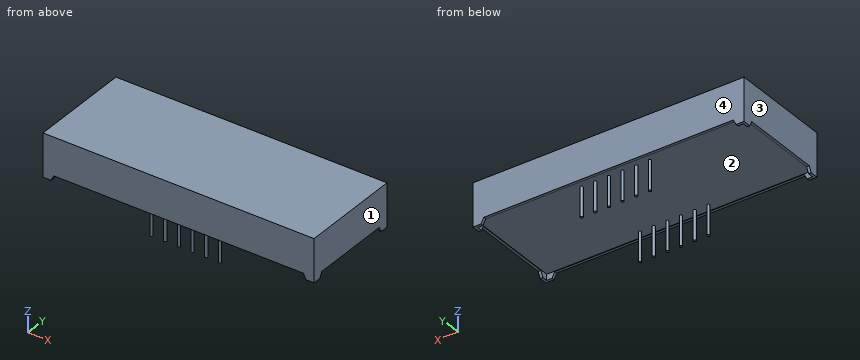
from build123d import *
from OCP.BRepFilletAPI import BRepFilletAPI_MakeChamfer

# Parameters (mm, degrees)
SKETCH1_W           = 50.4
SKETCH1_H           = 8
BOSS_EXTRUDE1_DEPTH = 19
CUT_EXTRUDE1_DEPTH  = 1
CHAMFER1_SIZE       = 0.5
CHAMFER1_SIZE_2     = 1
SKETCH3_W           = 49.4
SKETCH3_H           = 18
CUT_EXTRUDE2_DEPTH  = 0.1
SKETCH4_R           = 0.25
BOSS_EXTRUDE2_DEPTH = 5.5


with BuildPart() as part:
    # Sketch1 → Boss-Extrude1 (new body)
    with BuildSketch(Plane(origin=(0, 0, 0), x_dir=(1, 0, 0), z_dir=(0, 1, 0))):
        with Locations((25.2, 4)):
            Rectangle(SKETCH1_W, SKETCH1_H)
    extrude(amount=BOSS_EXTRUDE1_DEPTH)

    # Sketch2 → Cut-Extrude1 (cut)
    with BuildSketch(Plane(origin=(0, 0, -8), x_dir=(-1, 0, 0), z_dir=(0, 0, -1))):
        Polygon((-50.4, 17), (-49.9, 17), (-49.9, 18.5), (-48.4, 18.5), (-48.4, 19), (-2, 19), (-2, 18.5), (-0.5, 18.5), (-0.5, 17), (0, 17), (0, 2), (-0.5, 2), (-0.5, 0.5), (-2, 0.5), (-2, 0), (-48.4, 0), (-48.4, 0.5), (-49.9, 0.5), (-49.9, 2), (-50.4, 2), align=None)
    extrude(amount=-CUT_EXTRUDE1_DEPTH, mode=Mode.SUBTRACT)

    # Chamfer1
    chamfer1_edges_1 = [part.edges().sort_by_distance(p)[0] for p in [
        (50.15, 2, -8),
    ]]
    chamfer1_side_1 = [part.faces().sort_by_distance(p)[0] for p in [
        (50.15, 1.99, -8),
    ]]
    chamfer1_edges_2 = [part.edges().sort_by_distance(p)[0] for p in [
        (48.4, 0.25, -8),
    ]]
    chamfer1_side_2 = [part.faces().sort_by_distance(p)[0] for p in [
        (48.41, 0.25, -8),
    ]]
    chamfer1_edges_3 = [part.edges().sort_by_distance(p)[0] for p in [
        (2, 0.25, -8),
    ]]
    chamfer1_side_3 = [part.faces().sort_by_distance(p)[0] for p in [
        (1.99, 0.25, -8),
    ]]
    chamfer1_edges_4 = [part.edges().sort_by_distance(p)[0] for p in [
        (0.25, 2, -8),
    ]]
    chamfer1_side_4 = [part.faces().sort_by_distance(p)[0] for p in [
        (0.25, 2, -7.99),
    ]]
    chamfer1_edges_5 = [part.edges().sort_by_distance(p)[0] for p in [
        (2, 18.75, -8),
    ]]
    chamfer1_side_5 = [part.faces().sort_by_distance(p)[0] for p in [
        (1.99, 18.75, -8),
    ]]
    chamfer1_edges_6 = [part.edges().sort_by_distance(p)[0] for p in [
        (0.25, 17, -8),
    ]]
    chamfer1_side_6 = [part.faces().sort_by_distance(p)[0] for p in [
        (0.25, 17.01, -8),
    ]]
    chamfer1_edges_7 = [part.edges().sort_by_distance(p)[0] for p in [
        (48.4, 18.75, -8),
    ]]
    chamfer1_side_7 = [part.faces().sort_by_distance(p)[0] for p in [
        (48.41, 18.75, -8),
    ]]
    chamfer1_edges_8 = [part.edges().sort_by_distance(p)[0] for p in [
        (50.15, 17, -8),
    ]]
    chamfer1_side_8 = [part.faces().sort_by_distance(p)[0] for p in [
        (50.15, 17, -7.99),
    ]]
    chamfer1 = BRepFilletAPI_MakeChamfer(part.part.solid().wrapped)
    for e in chamfer1_edges_1:
        chamfer1.Add(CHAMFER1_SIZE - 0.0001, CHAMFER1_SIZE_2 - 0.0001, e.wrapped, chamfer1_side_1[0].wrapped)
    for e in chamfer1_edges_2:
        chamfer1.Add(CHAMFER1_SIZE - 0.0001, CHAMFER1_SIZE_2 - 0.0001, e.wrapped, chamfer1_side_2[0].wrapped)
    for e in chamfer1_edges_3:
        chamfer1.Add(CHAMFER1_SIZE - 0.0001, CHAMFER1_SIZE_2 - 0.0001, e.wrapped, chamfer1_side_3[0].wrapped)
    for e in chamfer1_edges_4:
        chamfer1.Add(CHAMFER1_SIZE_2 - 0.0001, CHAMFER1_SIZE - 0.0001, e.wrapped, chamfer1_side_4[0].wrapped)
    for e in chamfer1_edges_5:
        chamfer1.Add(CHAMFER1_SIZE - 0.0001, CHAMFER1_SIZE_2 - 0.0001, e.wrapped, chamfer1_side_5[0].wrapped)
    for e in chamfer1_edges_6:
        chamfer1.Add(CHAMFER1_SIZE - 0.0001, CHAMFER1_SIZE_2 - 0.0001, e.wrapped, chamfer1_side_6[0].wrapped)
    for e in chamfer1_edges_7:
        chamfer1.Add(CHAMFER1_SIZE - 0.0001, CHAMFER1_SIZE_2 - 0.0001, e.wrapped, chamfer1_side_7[0].wrapped)
    for e in chamfer1_edges_8:
        chamfer1.Add(CHAMFER1_SIZE_2 - 0.0001, CHAMFER1_SIZE - 0.0001, e.wrapped, chamfer1_side_8[0].wrapped)
    add(Compound.cast(chamfer1.Shape()), mode=Mode.REPLACE)  # a hair under: the kernel refuses the full size

    # Sketch3 → Cut-Extrude2 (cut)
    with BuildSketch(Plane(origin=(0, 0, -7), x_dir=(-1, 0, 0), z_dir=(0, 0, -1))):
        with Locations((-25.2, 9.5)):
            Rectangle(SKETCH3_W, SKETCH3_H)
    extrude(amount=-CUT_EXTRUDE2_DEPTH, mode=Mode.SUBTRACT)

    # Sketch4 → Boss-Extrude2 (add)
    with BuildSketch(Plane(origin=(0, 0, -6.9), x_dir=(-1, 0, 0), z_dir=(0, 0, -1))):
        with Locations(Location((-31.55, 17.12, 0), (0, 0, 180))):
            Circle(SKETCH4_R)
        with Locations(Location((-29.01, 17.12, 0), (0, 0, 180))):
            Circle(SKETCH4_R)
        with Locations(Location((-26.47, 17.12, 0), (0, 0, 180))):
            Circle(SKETCH4_R)
        with Locations(Location((-23.93, 17.12, 0), (0, 0, 180))):
            Circle(SKETCH4_R)
        with Locations(Location((-21.39, 17.12, 0), (0, 0, 180))):
            Circle(SKETCH4_R)
        with Locations(Location((-18.85, 17.12, 0), (0, 0, 180))):
            Circle(SKETCH4_R)
        with Locations(Location((-31.55, 1.88, 0), (0, 0, 180))):
            Circle(SKETCH4_R)
        with Locations(Location((-29.01, 1.88, 0), (0, 0, 180))):
            Circle(SKETCH4_R)
        with Locations(Location((-26.47, 1.88, 0), (0, 0, 180))):
            Circle(SKETCH4_R)
        with Locations(Location((-23.93, 1.88, 0), (0, 0, 180))):
            Circle(SKETCH4_R)
        with Locations(Location((-21.39, 1.88, 0), (0, 0, 180))):
            Circle(SKETCH4_R)
        with Locations(Location((-18.85, 1.88, 0), (0, 0, 180))):
            Circle(SKETCH4_R)
    extrude(amount=BOSS_EXTRUDE2_DEPTH)


solid = part.part
The model under review builds one solid part; all positions refer to its coordinate system, in mm. Face numbers are marked on the shaded views. Round coordinates to 2 decimals unless told otherwise and drop trailing zeros. Loops run counter-clockwise (first coordinate to the right, second up) from the corner with the lowest first, then second, coordinate; pieces in that order, holes last. Notation, with made-up numbers: M -10,33 L 37,33 A22 cw 37,44 Z; hole C 77,65.5 d10. An arc over 180 degrees is marked long. Answer as a JSON object with one key per item and string values.
Item 1: For line 1 along Z through (x, y) = (28, 14), list the stretches that pass through material, from the lowest coordinate up.
Check sheet entries:
{"line 1": "-6.9 to 0"}
Item 2: We need section A-A, the plane z = -8.5. State how many separate pieces and enclosed holes the cut face has, and give its area (3 significant figures).
Check sheet entries:
{"separate pieces": "12", "enclosed holes": "0", "area": "2.36 mm2"}
Item 3: We need section C-C, the plane y = 7.5. State the section outline as (x, z) points.
Check sheet entries:
{"outline": "M 0,-7 L 0.5,-7 L 0.5,-6.9 L 49.9,-6.9 L 49.9,-7 L 50.4,-7 L 50.4,0 L 0,0 Z"}
Item 4: The part is to be moulded in two halves that separate along X. For the marked faces 1, 2, 3 and 4, say which applies: +X half, -X half, draft (parallel to the pull), parting line (faces both ways), or undercut.
Check sheet entries:
{"face 1": "+X half", "face 2": "undercut", "face 3": "-X half", "face 4": "draft"}
Item 5: We need section B-B, the plane x = 16.5. State the section outline as (y, z) points, and give its area (3 significant figures).
Check sheet entries:
{"outline": "M 0,-7 L 0.5,-7 L 0.5,-6.9 L 18.5,-6.9 L 18.5,-7 L 19,-7 L 19,0 L 0,0 Z", "area": "131 mm2"}
Item 6: Clearance check with flat-ended pins moving along their axes: P1, Ø0.6, axis at x = 25, y = 0, coming from the -Z side; P2, Ø0.5, axis at x = 1, y = 0.5, coming from the -Z side; P3, Ø3, axis at x = 33.5, y = 10.5, coming from the -Z side. State where each tip first meets the part, or that it passes through.
Check sheet entries:
{"P1": "z = -7", "P2": "z = -8", "P3": "z = -6.9"}
